```python
from build123d import *

# Parameters (mm, degrees)
SKETCH1_R            = 5.25
BOSS_EXTRUDE1_DEPTH  = 8
BOSS_EXTRUDE2_DEPTH  = 10
LPATTERN1_COUNT      = 2
LPATTERN1_PITCH      = 50
MIRROR1_COPY_1_DEPTH = 10
CUT_EXTRUDE1_START   = -5
SKETCH3_R            = 15
CUT_EXTRUDE1_DEPTH   = 50


with BuildPart() as part:
    # Sketch1 → Boss-Extrude1 (new body)
    with BuildSketch(Plane.XY):
        with BuildLine():
            Line((105, 0), (105, 60))
            Line((105, 60), (95, 60))
            Line((95, 60), (95, 22.5))
            Line((95, 22.5), (82.5, 10))
            Line((82.5, 10), (67.5, 10))
            Line((67.5, 10), (55, 22.5))
            Line((55, 22.5), (55, 60))
            Line((55, 60), (45, 60))
            Line((45, 60), (45, 22.5))
            Line((45, 22.5), (32.5, 10))
            Line((32.5, 10), (20, 10))
            Line((20, 10), (7.5, 22.5))
            Line((7.5, 22.5), (7.5, 35))
            ThreePointArc((7.5, 35), (0, 42.5), (-7.5, 35))
            Line((-7.5, 35), (-7.5, 0))
            Line((-7.5, 0), (105, 0))
        make_face()
        Polygon((45, 15.428932188), (45, 10), (39.571067812, 10), align=None, mode=Mode.SUBTRACT)
        Polygon((60.428932188, 10), (55, 10), (55, 15.428932188), align=None, mode=Mode.SUBTRACT)
        Polygon((95, 15.428932188), (95, 10), (89.571067812, 10), align=None, mode=Mode.SUBTRACT)
        with Locations((0, 35)):
            Circle(SKETCH1_R, mode=Mode.SUBTRACT)
        Polygon((7.5, 15.428932188), (12.928932188, 10), (7.5, 10), align=None, mode=Mode.SUBTRACT)
    boss_extrude1 = extrude(amount=BOSS_EXTRUDE1_DEPTH)

    # Sketch2 → Boss-Extrude2 (add)
    with BuildSketch(Plane(origin=(45, 0, 0), x_dir=(0, 0, -1), z_dir=(1, 0, 0))):
        Polygon((7.5, 4.166666667), (0, 8.333333333), (0, 0), (7.5, 0), align=None)
    boss_extrude2 = extrude(amount=BOSS_EXTRUDE2_DEPTH)

    # LPattern1: Boss-Extrude2 ×2
    with Locations(*[(i * LPATTERN1_PITCH, 0, 0) for i in range(1, LPATTERN1_COUNT)]):
        add(boss_extrude2)

    # Mirror1: Boss-Extrude1, Boss-Extrude2 across plane
    add(boss_extrude1.mirror(Plane(origin=(55, 0, -7.5), x_dir=(1, 0, 0), z_dir=(0, 0, 1))))
    add(boss_extrude2.mirror(Plane(origin=(55, 0, -7.5), x_dir=(1, 0, 0), z_dir=(0, 0, 1))))

    # Mirror1 copy 1 sketch → Mirror1 copy 1 (add)
    with BuildSketch(Plane(origin=(95, 0, -15), x_dir=(0, 0, 1), z_dir=(1, 0, 0))):
        Polygon((7.5, -4.166666667), (0, -8.333333333), (0, 0), (7.5, 0), align=None)
    extrude(amount=MIRROR1_COPY_1_DEPTH)

    # Sketch3 → Cut-Extrude1 (cut)
    with BuildSketch(Plane(origin=(55, 0, 0), x_dir=(0, 0, -1), z_dir=(1, 0, 0)).offset(CUT_EXTRUDE1_START)):
        with Locations((7.5, 60)):
            Circle(SKETCH3_R)
    extrude(amount=CUT_EXTRUDE1_DEPTH, mode=Mode.SUBTRACT)


solid = part.part
```
Design review of the part built by this model. Coordinates are the model's own, in mm. A direction names the side the tool comes from. Give positions to 0.01 mm unless a question says otherwise; leave off trailing zeros. Write each loop counter-clockwise with the first axis right and the second up, starting at its lowest first coordinate (ties: lowest second). Pieces come first, ordered by that corner, then holes.
(1) Mouldability with a two-part tool opening along X and no side actions: class faces 1 (the face through (48, 24, 8)), 2 (the face through (-7.5, 18, -19)), 3 (the face through (55, 13, -19)) as +X half, -X half, draft (parallel to the pull), parting line (faces both ways), or undercut.
Checked values:
face 1: draft
face 2: -X half
face 3: undercut
(2) Wall thickness on line 1 along X through (y, z) = (23, 5); line 2 along Z through (x, y) = (49, 8.5); line 3 along X through (y, z) = (19, -21.5): over which ranges is each line inside the solid? List them lowest first.
Checked values:
line 1: x = -7.5 to 7.5, 45 to 55, 95 to 105
line 2: z = -23 to -15, 0 to 8
line 3: x = -7.5 to 11, 41.5 to 58.5, 91.5 to 105
(3) Add section B-B (x = 0). Give the boundary of the cut face in (y, z), and give its area (3 significant figures).
Checked values:
outline: (0, -23) - (29.75, -23) - (29.75, -15) - (0, -15) - close; (0, 0) - (29.75, 0) - (29.75, 8) - (0, 8) - close; (40.25, -23) - (42.5, -23) - (42.5, -15) - (40.25, -15) - close; (40.25, 0) - (42.5, 0) - (42.5, 8) - (40.25, 8) - close
area: 512 mm2
(4) Add section D-D (z = -3). Give the boundary of the cut face in (x, y), and give its area (3 significant figures).
Checked values:
outline: (45, 0) - (55, 0) - (55, 6.67) - (45, 6.67) - close; (95, 0) - (105, 0) - (105, 6.67) - (95, 6.67) - close
area: 133 mm2
(5) Add section A-A (y = 19). Give the boundary of the cut face in (x, z).
Checked values:
outline: (-7.5, -23) - (11, -23) - (11, -15) - (-7.5, -15) - close; (-7.5, 0) - (11, 0) - (11, 8) - (-7.5, 8) - close; (41.5, -23) - (58.5, -23) - (58.5, -15) - (41.5, -15) - close; (41.5, 0) - (58.5, 0) - (58.5, 8) - (41.5, 8) - close; (91.5, -23) - (105, -23) - (105, -15) - (91.5, -15) - close; (91.5, 0) - (105, 0) - (105, 8) - (91.5, 8) - close
(6) Tool access review of faces 4 (the face through (95, 37, -19)), 5 (the face through (102, 60, 4)), 6 (the face through (99.93, 6.22, -11.2)): name each direction out of +Z, -Z, +X, -X, +Y, -Y from which nothing blocks a thin tool from reaching the whole face with its end or side.
Checked values:
face 4: +Z, -Z, +Y
face 5: +Z, -Z, +X, -X, +Y
face 6: +X, -X, +Y
(7) Clearance check with flat-ended pins moving along their axes: pin 1 Ø12 at (y, z) = (43.5, -19) entering from -X; pin 2 Ø10 at (x, z) = (63, 0) entering from +Y; pin 3 Ø10 at (x, z) = (5.5, -14.5) entering from +Y. State where each tip first meets the part, or that it passes through.
Checked values:
pin 1: stops at x = -7.07
pin 2: stops at y = 19.5
pin 3: stops at y = 42.48
(8) Add section C-C (y = 5.5). Give the boundary of the cut face in (x, z).
Checked values:
outline: (-7.5, -23) - (105, -23) - (105, -9.9) - (95, -9.9) - (95, -15) - (55, -15) - (55, -9.9) - (45, -9.9) - (45, -15) - (-7.5, -15) - close; (-7.5, 0) - (45, 0) - (45, -5.1) - (55, -5.1) - (55, 0) - (95, 0) - (95, -5.1) - (105, -5.1) - (105, 8) - (-7.5, 8) - close
